The listing builds one solid part. Answer for the finished solid, in the listing's coordinates (mm). Face numbers are marked on the shaded views. A direction names the side the tool comes from. Coordinates: 2 decimals unless noted, no trailing zeros. Order: outer loops, then holes, each group sorted by start corner. A loop starts at its lowest first (then second) coordinate and runs counter-clockwise, first axis right, second up. Notation, with made-up numbers: (69, 69.25) -> (122, 69.25) arc R24 cw to (122, 85.25) -> close; hole circle Ø3 at (44, 53.5). An arc over 180 degrees is marked (long way). One line per question, with ' | ' between items.
from build123d import *

# Parameters (mm, degrees)
SKETCH1_R           = 50
BOSS_EXTRUDE1_DEPTH = 18
SKETCH2_R           = 4.057438755
BOSS_EXTRUDE2_DEPTH = 22
DOME1_FACE_RADIUS   = 4.057438755
DOME1_HEIGHT        = 3
DOME2_FACE_RADIUS   = 4.057438755
DOME2_HEIGHT        = 3
DOME3_FACE_RADIUS   = 4.057438755
DOME3_HEIGHT        = 3
DOME4_FACE_RADIUS   = 4.057438755
DOME4_HEIGHT        = 3


with BuildPart() as part:
    # Sketch1 → Boss-Extrude1 (new body)
    with BuildSketch(Plane(origin=(0, 0, 0), x_dir=(1, 0, 0), z_dir=(0, 1, 0))):
        Polygon((-27.487628691, 51.582330048), (-55.910904013, 17.03752672), (-51.582330048, -27.487628691), (-17.03752672, -55.910904013), (27.487628691, -51.582330048), (55.910904013, -17.03752672), (51.582330048, 27.487628691), (17.03752672, 55.910904013), align=None)
        Circle(SKETCH1_R, mode=Mode.SUBTRACT)
    extrude(amount=BOSS_EXTRUDE1_DEPTH)

    # Sketch2 → Boss-Extrude2 (add)
    with BuildSketch(Plane(origin=(0, 18, 0), x_dir=(1, 0, 0), z_dir=(0, 1, 0))):
        with Locations((-51.709884221, 15.757365217)):
            Circle(SKETCH2_R)
        with Locations((15.757365217, 51.709884221)):
            Circle(SKETCH2_R)
        with Locations((51.709884221, -15.757365217)):
            Circle(SKETCH2_R)
        with Locations((-15.757365217, -51.709884221)):
            Circle(SKETCH2_R)
    extrude(amount=BOSS_EXTRUDE2_DEPTH)

    # Dome1: a dome of height H over a round flat face of radius A is a cap of a sphere of radius (A * A + H * H) / (2 * H)
    dome1_r = (DOME1_FACE_RADIUS * DOME1_FACE_RADIUS + DOME1_HEIGHT * DOME1_HEIGHT) / (2 * DOME1_HEIGHT)
    dome1_base = Plane((-51.709884221, 40, -15.757365217), z_dir=(0, 1, 0))
    with Locations(dome1_base.offset(DOME1_HEIGHT - dome1_r)):
        dome1_ball = Sphere(dome1_r, mode=Mode.PRIVATE)
    add(split(dome1_ball, bisect_by=dome1_base, keep=Keep.TOP, mode=Mode.PRIVATE))

    # Dome2: a dome of height H over a round flat face of radius A is a cap of a sphere of radius (A * A + H * H) / (2 * H)
    dome2_r = (DOME2_FACE_RADIUS * DOME2_FACE_RADIUS + DOME2_HEIGHT * DOME2_HEIGHT) / (2 * DOME2_HEIGHT)
    dome2_base = Plane((15.757365217, 40, -51.709884221), z_dir=(0, 1, 0))
    with Locations(dome2_base.offset(DOME2_HEIGHT - dome2_r)):
        dome2_ball = Sphere(dome2_r, mode=Mode.PRIVATE)
    add(split(dome2_ball, bisect_by=dome2_base, keep=Keep.TOP, mode=Mode.PRIVATE))

    # Dome3: a dome of height H over a round flat face of radius A is a cap of a sphere of radius (A * A + H * H) / (2 * H)
    dome3_r = (DOME3_FACE_RADIUS * DOME3_FACE_RADIUS + DOME3_HEIGHT * DOME3_HEIGHT) / (2 * DOME3_HEIGHT)
    dome3_base = Plane((51.709884221, 40, 15.757365217), z_dir=(0, 1, 0))
    with Locations(dome3_base.offset(DOME3_HEIGHT - dome3_r)):
        dome3_ball = Sphere(dome3_r, mode=Mode.PRIVATE)
    add(split(dome3_ball, bisect_by=dome3_base, keep=Keep.TOP, mode=Mode.PRIVATE))

    # Dome4: a dome of height H over a round flat face of radius A is a cap of a sphere of radius (A * A + H * H) / (2 * H)
    dome4_r = (DOME4_FACE_RADIUS * DOME4_FACE_RADIUS + DOME4_HEIGHT * DOME4_HEIGHT) / (2 * DOME4_HEIGHT)
    dome4_base = Plane((-15.757365217, 40, 51.709884221), z_dir=(0, 1, 0))
    with Locations(dome4_base.offset(DOME4_HEIGHT - dome4_r)):
        dome4_ball = Sphere(dome4_r, mode=Mode.PRIVATE)
    add(split(dome4_ball, bisect_by=dome4_base, keep=Keep.TOP, mode=Mode.PRIVATE))


solid = part.part
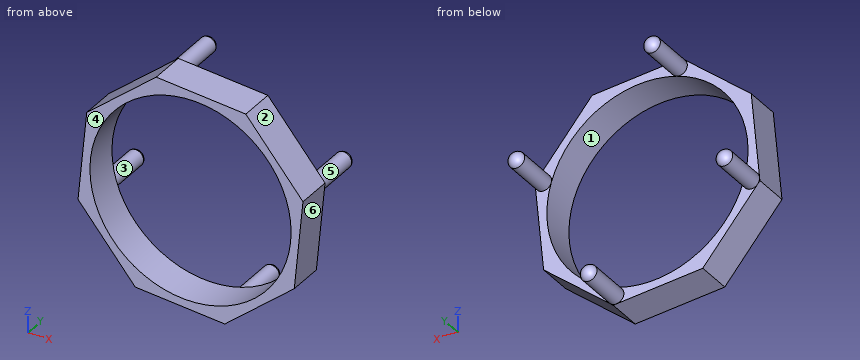
Item 1: Section A-A, the plane y = 8 is taken. Give the vertices of the cut face in (x, z).
Computed values:
outline: (-55.91, -17.04) -> (-27.49, -51.58) -> (17.04, -55.91) -> (51.58, -27.49) -> (55.91, 17.04) -> (27.49, 51.58) -> (-17.04, 55.91) -> (-51.58, 27.49) -> close; hole circle Ø100 at (0, 0)
Item 2: Each of these flat-tipped pins is pushed along its axis until it touches: pin 1 Ø10 at (y, z) = (28.5, 25) entering from -X; pin 2 Ø4 at (x, y) = (-22, 4.5) entering from -Z; pin 3 Ø12.5 at (x, z) = (36, 34.5) entering from +Y; pin 4 Ø3 at (y, z) = (34, 15.5) entering from -X. Where does it stop, or does it pass through?
Computed values:
pin 1: passes through | pin 2: stops at z = -52.31 | pin 3: stops at y = 18 | pin 4: stops at x = 47.65
Item 3: Section C-C, the plane x = 41 is taken. Give the vertices of the cut face in (y, z), plus the area to 3 significant figures.
Computed values:
outline: (0, -36.19) -> (18, -36.19) -> (18, -28.62) -> (0, -28.62) -> close; (0, 28.62) -> (18, 28.62) -> (18, 35.16) -> (0, 35.16) -> close | area: 254 mm^2
Item 4: Determine the mould class of the marked faces 1, 2, 3 and 4 for opening direction Z: pulls with the +Z half, pulls with the -Z half, needs draft (parallel to the pull), parting line crosses it, or undercut.
Computed values:
face 1: undercut | face 2: pulls with the +Z half | face 3: parting line crosses it | face 4: needs draft
Item 5: Section B-B, the plane z = 0 is taken. Give the vertices of the cut face in (x, y), plus the area to 3 significant figures.
Computed values:
outline: (-54.25, 0) -> (-50, 0) -> (-50, 18) -> (-54.25, 18) -> close; (50, 0) -> (54.25, 0) -> (54.25, 18) -> (50, 18) -> close | area: 153 mm^2
Item 6: Find the intervals of material crossed by L1, parallel to Z at x = 0, y = 12.5; L2, parallel to Z at x = 29.5, y = 15; L3, parallel to Y at x = 50, z = -11, in increasing order.
Computed values:
L1: z = -54.25 to -50, 50 to 54.25 | L2: z = -45.66 to -40.37, 40.37 to 49.14 | L3: y = 0 to 18
Item 7: For the marked faces 5 and 6, determine the directions among +Z, -Z, +X, -X, +Y, -Y from which every point of the face is accessible in a straight line to the end or side of a thin tool.
Computed values:
face 5: +Y | face 6: -Z, +X, +Y, -Y
